```python
from build123d import *

# Parameters (mm, degrees)
SKETCH1_W                = 180
SKETCH1_H                = 110
BOSS_EXTRUDE1_DEPTH      = 50
BOSS_EXTRUDE2_DEPTH      = 180
CUT_EXTRUDE1_DEPTH       = 146.344418537
BOSS_EXTRUDE5_DEPTH      = 10
BOSS_EXTRUDE5_DEPTH_BACK = 10
SKETCH5_R                = 5


with BuildPart() as part:
    # Sketch1 → Boss-Extrude1 (new body)
    with BuildSketch(Plane(origin=(0, 0, 0), x_dir=(1, 0, 0), z_dir=(0, 1, 0))):
        Rectangle(SKETCH1_W, SKETCH1_H)
    extrude(amount=BOSS_EXTRUDE1_DEPTH)

    # Sketch2 → Boss-Extrude2 (add)
    with BuildSketch(Plane.ZY.offset(90)):
        with BuildLine():
            Line((-55, 0), (55, 0))
            ThreePointArc((55, 0), (0, -50), (-55, 0))
        make_face()
    extrude(amount=-BOSS_EXTRUDE2_DEPTH)

    # Sketch3 → Cut-Extrude1 (cut, through all)
    with BuildSketch(Plane(origin=(0, 50, 0), x_dir=(1, 0, 0), z_dir=(0, 1, 0))):
        Polygon((-49.118803686, -55), (-90, 15.808309091), (-90, -55), align=None)
    cut_extrude1 = extrude(amount=-CUT_EXTRUDE1_DEPTH, mode=Mode.SUBTRACT)

    # Mirror1: Cut-Extrude1 across plane
    add(cut_extrude1.mirror(Plane(origin=(0, 0, 0), x_dir=(0, 0, 1), z_dir=(1, 0, 0))), mode=Mode.SUBTRACT)

    # Sketch5 → Boss-Extrude5 (add, two sides: drawn at the far end of the back side and taken through both)
    with BuildSketch(Plane(origin=(0, 0, -55), x_dir=(-1, 0, 0), z_dir=(0, 0, -1)).offset(-BOSS_EXTRUDE5_DEPTH_BACK)):
        Circle(SKETCH5_R)
    extrude(amount=BOSS_EXTRUDE5_DEPTH + BOSS_EXTRUDE5_DEPTH_BACK)

    # Sketch4 → Revolve1 (revolve)
    with BuildSketch(Plane(origin=(-60.654801368, 0, 35.019065898), x_dir=(0.49999999999999495, 0, 0.8660254037844417), z_dir=(-0.8660254037844417, 0, 0.49999999999999495))):
        with BuildLine():
            ThreePointArc((-20.965161058, 42.942576489), (4.034838942, 17.942576489), (-20.965161058, -7.057423511))
            Line((-20.965161058, -7.057423511), (-20.965161058, 42.942576489))
        make_face()
    revolve1 = revolve(axis=Axis((-71.137381897, 42.942576489, 16.862703827), (0, -1, 0)))

    # Mirror2: Revolve1 across plane
    add(revolve1.mirror(Plane(origin=(0, 0, 0), x_dir=(0, 0, 1), z_dir=(1, 0, 0))))


solid = part.part
```
Design review of the part built by this model. Coordinates are the model's own, in mm. A direction names the side the tool comes from. Give positions to 0.01 mm unless a question says otherwise; leave off trailing zeros. Write each loop counter-clockwise with the first axis right and the second up, starting at its lowest first coordinate (ties: lowest second). Pieces come first, ordered by that corner, then holes.
(1) Add section B-B (y = 34). Give the boundary of the cut face in (x, z), and give its area (3 significant figures).
Checked values:
outline: (-90, -55) - (90, -55) - (90, -15.81) - (80.72, 0.27) arc R19.16 ccw to (61.56, 33.46) - (49.12, 55) - (-49.12, 55) - (-61.56, 33.46) arc R19.16 ccw to (-80.72, 0.27) - (-90, -15.81) - close
area: 18,100 mm2
(2) Add section D-D (z = 2.5). Give the boundary of the cut face in (x, y).
Checked values:
outline: (-79.43, -49.94) - (79.43, -49.94) - (79.43, -0.76) arc R20.46 ccw to (79.43, 36.65) - (79.43, 50) - (-79.43, 50) - (-79.43, 36.65) arc R20.46 ccw to (-79.43, -0.76) - close
(3) Tool access review of faces 1 (the face through (1.08, -4.88, -59.57)), 2 (the face through (-90, 2, -35)), 3 (the face through (90, 2, -35)): name each direction out of +Z, -Z, +X, -X, +Y, -Y from which nothing blocks a thin tool from reaching the whole face with its end or side.
Checked values:
face 1: -Z
face 2: -Z, -X, +Y, -Y
face 3: -Z, +X, +Y, -Y
(4) Clearance check with flat-ended pins moving along their axes: pin 1 Ø10 at (y, z) = (-31.5, 37) entering from +X; pin 2 Ø8 at (x, z) = (-55, -12) entering from -Y; pin 3 Ø8 at (x, z) = (11, 3.5) entering from -Y; pin 4 Ø15 at (x, y) = (-11, 24) entering from -Z. State where each tip first meets the part, or that it passes through.
Checked values:
pin 1: stops at x = 62.4
pin 2: stops at y = -49.42
pin 3: stops at y = -50
pin 4: stops at z = -55
(5) Add section A-A (x = 0). Give the boundary of the cut face in (y, z).
Checked values:
outline: (-5, -65) - (5, -65) - (5, -55) - (50, -55) - (50, 55) - (0, 55) arc R55.25 ccw to (-5, -54.29) - close
(6) Add section C-C (z = 31). Give the boundary of the cut face in (x, y), and give its area (3 significant figures).
Checked values:
outline: (-62.98, -40.48) - (62.98, -40.48) - (62.98, -0.99) arc R20.62 ccw (long way) to (62.98, 36.88) - (62.98, 50) - (-62.98, 50) - (-62.98, 36.88) arc R20.62 ccw (long way) to (-62.98, -0.99) - close
area: 13,400 mm2
(7) Wall thickness on line 1 along X through (y, z) = (21.5, 39); line 2 along Z through (x, y) = (21.5, 19.5); line 3 along Y through (x, z) = (32.5, -1.5): over which ranges is each line inside the solid? List them lowest first.
Checked values:
line 1: x = -82.2 to -60.08, -58.36 to 58.36, 60.08 to 82.2
line 2: z = -55 to 55
line 3: y = -49.98 to 50
